Build history of the part. All positions in model axes, mm. A direction names the side the tool comes from. Give positions to 0.01 mm unless a question says otherwise; leave off trailing zeros. Loops run counter-clockwise (first coordinate to the right, second up) from the corner with the lowest first, then second, coordinate; pieces in that order, holes last. Notation, with made-up numbers: (49.5, 86.5) -> (72.5, 86.5) arc R24 cw to (72.5, 97.5) -> close; hole circle Ø4 at (2, -6). An arc over 180 degrees is marked (long way). Answer in a Markdown table with one row per item. Add a question column.
from build123d import *

# Parameters (mm, degrees)
SKIZZE1_R                        = 100
AUFSATZ_LINEAR_AUSTRAGEN1_DEPTH  = 15
AUFSATZ_LINEAR_AUSTRAGEN2_DEPTH  = 55
SCHNITT_LINEAR_AUSTRAGEN5_REACH  = 188.497
SKIZZE7_R                        = 15
SCHNITT_LINEAR_AUSTRAGEN6_DEPTH  = 10
SKIZZE10_R                       = 10
SCHNITT_LINEAR_AUSTRAGEN9_DEPTH  = 5
SCHNITT_LINEAR_START             = -5
SKIZZE11_R                       = 10
SCHNITT_LINEAR_AUSTRAGEN10_DEPTH = 5
SKIZZE12_R                       = 90
SKIZZE12_R_2                     = 84
SCHNITT_LINEAR_AUSTRAGEN11_DEPTH = 2.8
SKIZZE13_R                       = 5
SCHNITT_LINEAR_AUSTRAGEN12_DEPTH = 5
SKIZZE14_R                       = 12
SCHNITT_LINEAR_AUSTRAGEN13_DEPTH = 10


with BuildPart() as part:
    # Skizze1 → Aufsatz-Linear austragen1 (new body)
    with BuildSketch(Plane(origin=(0, 0, 0), x_dir=(1, 0, 0), z_dir=(0, 1, 0))):
        with Locations(Location((0, 0, 0), (0, 0, 270))):
            Circle(SKIZZE1_R)
    extrude(amount=AUFSATZ_LINEAR_AUSTRAGEN1_DEPTH)

    # Skizze2 → Aufsatz-Linear austragen2 (add)
    with BuildSketch(Plane(origin=(0, 15, 0), x_dir=(1, 0, 0), z_dir=(0, 1, 0))):
        Polygon((-26, -25), (-26, 25), (-26, 26), (-41, 26), (-41, -26), (-26, -26), align=None)
        Polygon((26, 26), (26, 25), (26, -25), (26, -26), (41, -26), (41, 26), align=None)
    extrude(amount=AUFSATZ_LINEAR_AUSTRAGEN2_DEPTH)

    # Schnitt-Linear austragen5: up to this face of the body (flat: up to its plane)
    schnitt_linear_austragen5_end = Plane(part.part.faces().sort_by_distance((41, 42.5, 0))[0])
    # Skizze3 → Schnitt-Linear austragen5 (cut, up to the picked face)
    with BuildSketch(Plane.ZY.offset(41), mode=Mode.PRIVATE) as schnitt_linear_austragen5_sk1:
        with BuildLine():
            Line((-26, 70), (-26, 44))
            ThreePointArc((-26, 44), (-18.384776279, 62.384776343), (9.1e-08, 70))
            Line((9.1e-08, 70), (-26, 70))
        make_face()
    schnitt_linear_austragen5_tool1 = split(extrude(schnitt_linear_austragen5_sk1.sketch, amount=-SCHNITT_LINEAR_AUSTRAGEN5_REACH, mode=Mode.PRIVATE), bisect_by=schnitt_linear_austragen5_end, keep=Keep.BOTH, mode=Mode.PRIVATE)
    # Skizze3 → Schnitt-Linear austragen5 (cut, up to the picked face)
    with BuildSketch(Plane.ZY.offset(41), mode=Mode.PRIVATE) as schnitt_linear_austragen5_sk2:
        with BuildLine():
            ThreePointArc((9.1e-08, 70), (18.384776343, 62.384776279), (26, 44))
            Line((26, 44), (26, 70))
            Line((26, 70), (9.1e-08, 70))
        make_face()
    schnitt_linear_austragen5_tool2 = split(extrude(schnitt_linear_austragen5_sk2.sketch, amount=-SCHNITT_LINEAR_AUSTRAGEN5_REACH, mode=Mode.PRIVATE), bisect_by=schnitt_linear_austragen5_end, keep=Keep.BOTH, mode=Mode.PRIVATE)
    add(schnitt_linear_austragen5_tool1.solids().sort_by(Axis((-41, 64.192434, -20.192434), (1, 0, 0)))[0], mode=Mode.SUBTRACT)
    add(schnitt_linear_austragen5_tool2.solids().sort_by(Axis((-41, 64.192434, 20.192434), (1, 0, 0)))[0], mode=Mode.SUBTRACT)

    # Skizze7 → Schnitt-Linear austragen6 (cut)
    with BuildSketch(Plane.ZY.offset(41)):
        with Locations((0, 44)):
            Circle(SKIZZE7_R)
    schnitt_linear_austragen6 = extrude(amount=-SCHNITT_LINEAR_AUSTRAGEN6_DEPTH, mode=Mode.SUBTRACT)

    # Skizze10 → Schnitt-Linear austragen9 (cut)
    with BuildSketch(Plane(origin=(0, 15, 0), x_dir=(1, 0, 0), z_dir=(0, 1, 0))):
        with Locations(Location((0, 0, 0), (0, 0, 270))):
            Circle(SKIZZE10_R)
    extrude(amount=-SCHNITT_LINEAR_AUSTRAGEN9_DEPTH, mode=Mode.SUBTRACT)

    # Skizze11 → Schnitt-Linear austragen10 (cut)
    with BuildSketch(Plane.XZ.offset(SCHNITT_LINEAR_START)):
        with Locations(Location((0, 0, 0), (0, 0, 90))):
            Circle(SKIZZE11_R)
    extrude(amount=SCHNITT_LINEAR_AUSTRAGEN10_DEPTH, mode=Mode.SUBTRACT)

    # Skizze12 → Schnitt-Linear austragen11 (cut)
    with BuildSketch(Plane.XZ):
        with Locations(Location((0, 0, 0), (0, 0, 270))):
            Circle(SKIZZE12_R)
        with Locations(Location((0, 0, 0), (0, 0, 270))):
            Circle(SKIZZE12_R_2, mode=Mode.SUBTRACT)
    extrude(amount=-SCHNITT_LINEAR_AUSTRAGEN11_DEPTH, mode=Mode.SUBTRACT)

    # Skizze13 → Schnitt-Linear austragen12 (cut)
    with BuildSketch(Plane.XZ.offset(-5)):
        with Locations(Location((0, 0, 0), (0, 0, 270))):
            Circle(SKIZZE13_R)
    extrude(amount=-SCHNITT_LINEAR_AUSTRAGEN12_DEPTH, mode=Mode.SUBTRACT)

    # Skizze14 → Schnitt-Linear austragen13 (cut)
    with BuildSketch(Plane(origin=(-26, 0, 0), x_dir=(0, 0, -1), z_dir=(1, 0, 0))):
        with Locations((0, 44)):
            Circle(SKIZZE14_R)
    schnitt_linear_austragen13 = extrude(amount=-SCHNITT_LINEAR_AUSTRAGEN13_DEPTH, mode=Mode.SUBTRACT)

    # Spiegeln1: Schnitt-Linear austragen6, Schnitt-Linear austragen13 across plane
    add(schnitt_linear_austragen6.mirror(Plane(origin=(0, 0, 0), x_dir=(0, 0, 1), z_dir=(1, 0, 0))), mode=Mode.SUBTRACT)
    add(schnitt_linear_austragen13.mirror(Plane(origin=(0, 0, 0), x_dir=(0, 0, 1), z_dir=(1, 0, 0))), mode=Mode.SUBTRACT)


solid = part.part
(1) Saw through at A-A, the plane x = 0. List the corners of the cut face in (y, z), then the cut area to 3 significant figures.
(2) Wall check: line 1 along X through (y, z) = (43, -12); line 2 along Z through (x, y) = (27.85, 44); line 3 along X through (y, z) = (43.5, -21). Give the ranges that are in metal, low to high. Write a range as from..to.
(3) Flat gauge pins, fed straight in: pin 1 Ø24 at (y, z) = (44.5, -2) entering from -X; pin 2 Ø12 at (x, z) = (0, 0) entering from +Y; pin 3 Ø4.5 at (x, y) = (32.5, 27.5) entering from +Z. Where does each tip first touch, or does it go through?
(4) 3-axis set-ups, long thin cutter, end or side, ignore diameter. For faces 1 (the cylindrical face through (36.07, 58.872, -1.953)), 2 (the flat face through (5, 10, 2)), 3 (the flat face through (26, 30, 0)), 4 (the cylindrical face through (25.23, 1.38, -80.12)): which of +Z, -Z, +X, -X, +Y, -Y reach the whole face in a straight line?
(5) Saw through at C-C, the plane z = 19. List the corners of the cut face in (x, y), then the cut area to 3 significant figures.
(6) Saw through at D-D, the plane x = 77.5. List the corners of the cut face in (y, z), then the cut area to 3 significant figures.
(7) Saw through at B-B, the plane y = 64. List the corners of the cut face in (x, z), then the cut area to 3 significant figures.
(8) Two-plate mould, pull along X, no slides. Class faces 5 (the cylindrical face through (9.76, 2.54, -2.17)), 6 (the flat face through (31, 54, -7)), 7 (the flat face through (-5, 5, 2)), 8 (the cylindrical face through (28.465, 32.285, 2.601)): released by +X, released by -X, zero draft, split by the parting line, or undercut.
Worked answers:
| question | item | result |
|---|---|---|
| 1 | outline | (0, -100) -> (15, -100) -> (15, -10) -> (10, -10) -> (10, -5) -> (5, -5) -> (5, -10) -> (0, -10) -> (0, -84) -> (2.8, -84) -> (2.8, -90) -> (0, -90) -> close; (0, 10) -> (5, 10) -> (5, 5) -> (10, 5) -> (10, 10) -> (15, 10) -> (15, 100) -> (0, 100) -> (0, 90) -> (2.8, 90) -> (2.8, 84) -> (0, 84) -> close |
| 1 | area | 2,720 mm^2 |
| 2 | line 1 | -31..-26, 26..31 |
| 2 | line 2 | -26..-12, 12..26 |
| 2 | line 3 | -41..-26, 26..41 |
| 3 | pin 1 | x = -31 |
| 3 | pin 2 | y = 10 |
| 3 | pin 3 | z = 26 |
| 4 | face 1 | +X |
| 4 | face 2 | +Y |
| 4 | face 3 | +Z, -Z, +Y |
| 4 | face 4 | -Y |
| 5 | outline | (-98.18, 0) -> (-87.97, 0) -> (-87.97, 2.8) -> (-81.82, 2.8) -> (-81.82, 0) -> (81.82, 0) -> (81.82, 2.8) -> (87.97, 2.8) -> (87.97, 0) -> (98.18, 0) -> (98.18, 15) -> (41, 15) -> (41, 61.75) -> (26, 61.75) -> (26, 15) -> (-26, 15) -> (-26, 61.75) -> (-41, 61.75) -> (-41, 15) -> (-98.18, 15) -> close |
| 5 | area | 4,310 mm^2 |
| 6 | outline | (0, -63.2) -> (15, -63.2) -> (15, 63.2) -> (0, 63.2) -> (0, 45.76) -> (2.8, 45.76) -> (2.8, 32.4) -> (0, 32.4) -> (0, -32.4) -> (2.8, -32.4) -> (2.8, -45.76) -> (0, -45.76) -> close |
| 6 | area | 1,820 mm^2 |
| 7 | outline | (-41, -16.61) -> (-26, -16.61) -> (-26, 16.61) -> (-41, 16.61) -> close; (26, -16.61) -> (41, -16.61) -> (41, 16.61) -> (26, 16.61) -> close |
| 7 | area | 997 mm^2 |
| 8 | face 5 | undercut |
| 8 | face 6 | released by +X |
| 8 | face 7 | undercut |
| 8 | face 8 | zero draft |
